The model under review builds one solid part; all positions refer to its coordinate system, in mm. Face numbers are marked on the shaded views. Round coordinates to 2 decimals unless told otherwise and drop trailing zeros. Order: outer loops, then holes, each group sorted by start corner. A loop starts at its lowest first (then second) coordinate and runs counter-clockwise, first axis right, second up. Notation, with made-up numbers: (74, -18.5) -> (85, -18.5) arc R13 cw to (85, 6.5) -> close; hole circle Ø9 at (0.25, -25). An arc over 180 degrees is marked (long way). Return JSON: item names as keys, results as strings. Group by question number.
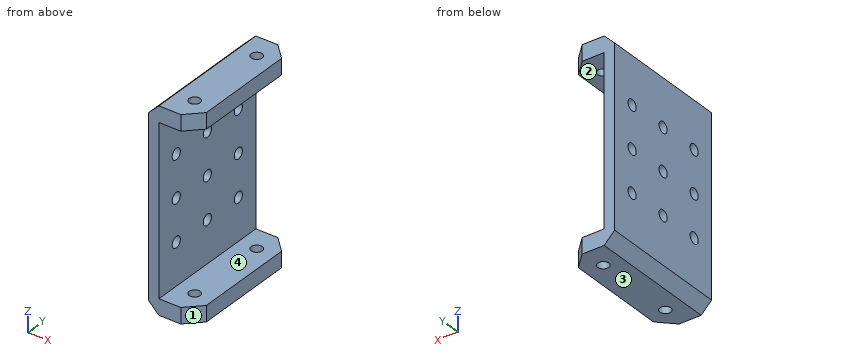
from build123d import *

# Parameters (mm, degrees)
SKETCH_1_W                  = 25
SKETCH_1_H                  = 38
EXTRUDE_1_DEPTH             = 9
CUT_EXTRUDE_1_DEPTH         = 47.368092477
HOLE_WIZARD_2_1_2_1_1_D     = 2.1
HOLE_WIZARD_2_1_2_1_1_DEPTH = 9
HOLE_WIZARD_2_1_2_1_2_D     = 2.1
HOLE_WIZARD_2_1_2_1_2_DEPTH = 9
HOLE_WIZARD_2_1_2_1_3_D     = 2.1
HOLE_WIZARD_2_1_2_1_3_DEPTH = 9
HOLE_WIZARD_2_1_2_1_4_D     = 2.1
HOLE_WIZARD_2_1_2_1_4_DEPTH = 3.007193387
CHAMFER_1_SIZE              = 2
SKETCH_12_R                 = 1.05
CUT_EXTRUDE_2_DEPTH         = 10
SKETCH_15_R                 = 1.05
CUT_EXTRUDE_3_DEPTH         = 10
CUT_EXTRUDE_4_DEPTH         = 47.368092478
CUT_EXTRUDE_5_DEPTH         = 47.368092477
CUT_EXTRUDE_5_DEPTH_BACK    = 47.368092477


with BuildPart() as part:
    # 草图1 → 凸台-拉伸1 (new body)
    with BuildSketch(Plane(origin=(0, 0, 0), x_dir=(0, -1, 0), z_dir=(-1, 0, 0))):
        with Locations((-12.5, 19)):
            Rectangle(SKETCH_1_W, SKETCH_1_H)
    extrude(amount=-EXTRUDE_1_DEPTH)

    # 草图2 → 切除-拉伸1 (cut, through all)
    with BuildSketch(Plane(origin=(0, 25, 0), x_dir=(-1, 0, 0), z_dir=(0, 1, 0))):
        Polygon((-9, 3), (-4, 3), (-3.996522166, 5.080336705), (-3.996522166, 33.000000217), (-3.996522166, 34.992806613), (-9, 34.992806613), align=None)
    extrude(amount=-CUT_EXTRUDE_1_DEPTH, mode=Mode.SUBTRACT)

    # Ø2.1 (2.1) 直径孔1
    with Locations(Plane.ZY):
        with Locations((11, 4.5)):
            Hole(HOLE_WIZARD_2_1_2_1_1_D / 2, depth=HOLE_WIZARD_2_1_2_1_1_DEPTH)

    # Ø2.1 (2.1) 直径孔2
    with Locations(Plane.ZY):
        with Locations((19, 4.5)):
            Hole(HOLE_WIZARD_2_1_2_1_2_D / 2, depth=HOLE_WIZARD_2_1_2_1_2_DEPTH)

    # Ø2.1 (2.1) 直径孔3
    with Locations(Plane.ZY):
        with Locations((27, 4.5), (27, 12.5), (27, 20.5), (11, 12.5), (11, 20.5), (19, 20.5), (19, 12.5)):
            Hole(HOLE_WIZARD_2_1_2_1_3_D / 2, depth=HOLE_WIZARD_2_1_2_1_3_DEPTH)

    # Ø2.1 (2.1) 直径孔4
    with Locations(Plane(origin=(0, 0, 34.992806613), x_dir=(-1, 0, 0), z_dir=(0, 0, -1))):
        with Locations((-5.5, 4.5), (-5.5, 20.5)):
            Hole(HOLE_WIZARD_2_1_2_1_4_D / 2, depth=HOLE_WIZARD_2_1_2_1_4_DEPTH)

    # 倒角1
    chamfer_1_edges = [part.edges().sort_by_distance(p)[0] for p in [
        (0, 12.5, 0),
        (0, 12.5, 38),
    ]]
    chamfer(chamfer_1_edges, length=CHAMFER_1_SIZE)

    # 草图12 → 切除-拉伸2 (cut)
    with BuildSketch(Plane.XY.offset(3)):
        with Locations(Location((5.5, 4.5, 0), (0, 0, 180))):
            Circle(SKETCH_12_R)
    extrude(amount=-CUT_EXTRUDE_2_DEPTH, mode=Mode.SUBTRACT)

    # 草图15 → 切除-拉伸3 (cut)
    with BuildSketch(Plane.XY.offset(3)):
        with Locations(Location((5.5, 20.5, 0), (0, 0, 180))):
            Circle(SKETCH_15_R)
    extrude(amount=-CUT_EXTRUDE_3_DEPTH, mode=Mode.SUBTRACT)

    # 草图16 → 切除-拉伸4 (cut, through all)
    with BuildSketch(Plane.XZ):
        Polygon((3.996522166, 34.992806613), (1.996522166, 34.992806613), (2, 3), (4, 3), align=None)
    extrude(amount=-CUT_EXTRUDE_4_DEPTH, mode=Mode.SUBTRACT)

    # 草图17 → 切除-拉伸5 (cut, two sides: drawn at the far end of the back side and taken through both)
    with BuildSketch(Plane.XY.offset(38).offset(-CUT_EXTRUDE_5_DEPTH_BACK)):
        Polygon((9, 22.2), (6.2, 25), (9, 25), align=None)
        Polygon((9, 0), (9, 2.8), (6.2, 0), align=None)
    extrude(amount=CUT_EXTRUDE_5_DEPTH + CUT_EXTRUDE_5_DEPTH_BACK, mode=Mode.SUBTRACT)


solid = part.part
Item 1: Consider section B-B on y = 16. State the section outline as (x, z) points, plus the area to 3 significant figures.
Item 2: Consider section A-A on z = 19. State the section outline as (x, y) points, plus the area to 3 significant figures.
Item 3: The part is to be moulded in two halves that separate along Z. For the marked faces 1, 2, 3 and 4, say which applies: +Z half, -Z half, draft (parallel to the pull), parting line (faces both ways), or undercut.
Item 4: Consider section C-C on x = 0.75. Give the number of separate pieces and of enclosed holes in the cut face, plus the area to 3 significant figures.
Item 5: Wall thickness on line 1 along Y through (x, z) = (0.8, 27); line 2 along Y through (x, z) = (5.5, 1); line 3 along Z through (x, y) = (2.25, 8): over which ranges is each line inside the solid? List them lowest first.
Item 6: Insertion check: pin 1 Ø2.5 at (y, z) = (4.5, 27) entering from +X. The pin has a flat end and moves straight along its axis. Give the tip position at first contact, or say it passes through.
Values:
{
 "1": {"outline": "(0, 2) -> (2, 0) -> (9, 0) -> (9, 3) -> (2, 3) -> (2, 34.99) -> (9, 34.99) -> (9, 38) -> (2, 38) -> (0, 36) -> close", "area": "114 mm^2"},
 "2": {"outline": "(0, 0) -> (2, 0) -> (2, 3.45) -> (0, 3.45) -> close; (0, 5.55) -> (2, 5.55) -> (2, 11.45) -> (0, 11.45) -> close; (0, 13.55) -> (2, 13.55) -> (2, 19.45) -> (0, 19.45) -> close; (0, 21.55) -> (2, 21.55) -> (2, 25) -> (0, 25) -> close", "area": "37.4 mm^2"},
 "3": {"face 1": "draft", "face 2": "undercut", "face 3": "-Z half", "face 4": "undercut"},
 "4": {"separate pieces": "1", "enclosed holes": "9", "area": "856 mm^2"},
 "5": {"line 1": "0 to 3.45, 5.55 to 11.45, 13.55 to 19.45, 21.55 to 25", "line 2": "0 to 3.45, 5.55 to 19.45, 21.55 to 25", "line 3": "0 to 3, 34.99 to 38"},
 "6": {"pin 1": "x = 2"}
}
